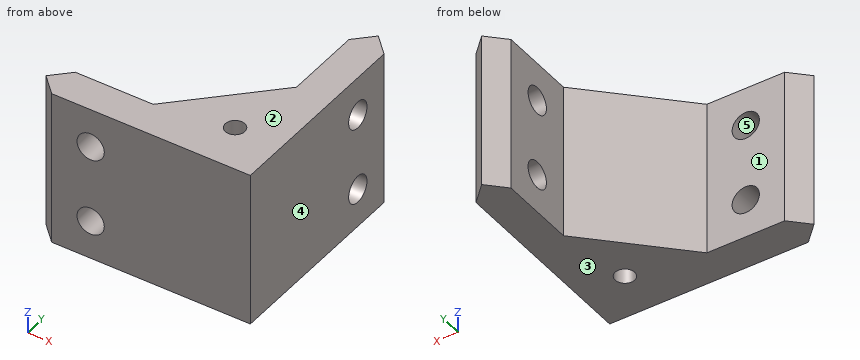
from build123d import *

# Parameters (mm, degrees)
BOSS_EXTRUDE1_DEPTH = 40
SKETCH2_R           = 3.5
CUT_EXTRUDE1_DEPTH  = 84.3366666
SKETCH3_R           = 3.5
CUT_EXTRUDE2_DEPTH  = 40
CHAMFER1_SIZE       = 5
SKETCH4_R           = 2.5
CUT_EXTRUDE3_DEPTH  = 40


with BuildPart() as part:
    # Sketch1 → Boss-Extrude1 (new body)
    with BuildSketch(Plane.XY):
        Polygon((0, 56), (0, 0), (-56, 0), (-56, 9), (-31, 9), (-9, 31), (-9, 56), align=None)
    extrude(amount=BOSS_EXTRUDE1_DEPTH)

    # Sketch2 → Cut-Extrude1 (cut, through all)
    with BuildSketch(Plane.ZY.offset(9)):
        with Locations((10, 41)):
            Circle(SKETCH2_R)
        with Locations((30, 41)):
            Circle(SKETCH2_R)
    extrude(amount=-CUT_EXTRUDE1_DEPTH, mode=Mode.SUBTRACT)

    # Sketch3 → Cut-Extrude2 (cut)
    with BuildSketch(Plane(origin=(0, 9, 0), x_dir=(1, 0, 0), z_dir=(0, 1, 0))):
        with Locations(Location((-41, -10, 0), (0, 0, 270))):
            Circle(SKETCH3_R)
        with Locations(Location((-41, -30, 0), (0, 0, 270))):
            Circle(SKETCH3_R)
    extrude(amount=-CUT_EXTRUDE2_DEPTH, mode=Mode.SUBTRACT)

    # Chamfer1
    # the kernel refuses this chamfer: 5 mm, written as the material it takes off along each edge
    with BuildSketch(Plane(origin=(-56, 0, -12.85841494), x_dir=(0.9996219169112968, -0.027495876610586254, 0), z_dir=(0, 0, 1)), Plane(origin=(-56, 9, -12.85841494), x_dir=(-0.027495876610586317, -0.9996219169112968, 0), z_dir=(0, 0, 1))) as chamfer1_piece_1:
        Polygon((CHAMFER1_SIZE * 0.999621916911, CHAMFER1_SIZE * 0.0274958766106), (-CHAMFER1_SIZE * 0.0274958766106, CHAMFER1_SIZE * 0.999621916911), (0, 0), align=None)
    extrude(amount=65.71682988, mode=Mode.SUBTRACT)
    with BuildSketch(Plane(origin=(0, 56, -12.85841494), x_dir=(0.02749587661058641, -0.9996219169112968, 0), z_dir=(0, 0, 1)), Plane(origin=(-9, 56, -12.85841494), x_dir=(0.9996219169112968, 0.027495876610586317, 0), z_dir=(0, 0, 1))) as chamfer1_piece_2:
        Polygon((CHAMFER1_SIZE * 0.999621916911, -CHAMFER1_SIZE * 0.0274958766106), (-CHAMFER1_SIZE * 0.0274958766106, -CHAMFER1_SIZE * 0.999621916911), (0, 0), align=None)
    extrude(amount=65.71682988, mode=Mode.SUBTRACT)

    # Sketch4 → Cut-Extrude3 (cut)
    with BuildSketch(Plane(origin=(0, 0, 0), x_dir=(-1, 0, 0), z_dir=(0, 0, -1))):
        with Locations((12, 12)):
            Circle(SKETCH4_R)
    extrude(amount=-CUT_EXTRUDE3_DEPTH, mode=Mode.SUBTRACT)


solid = part.part
The listing builds one solid part. Answer for the finished solid, in the listing's coordinates (mm). Face numbers are marked on the shaded views. A direction names the side the tool comes from. Give positions to 0.01 mm unless a question says otherwise; leave off trailing zeros. Loops run counter-clockwise (first coordinate to the right, second up) from the corner with the lowest first, then second, coordinate; pieces in that order, holes last. Notation, with made-up numbers: (-34.5, 64) - (8.5, 64) arc R30 ccw to (8.5, 90) - close; hole circle Ø2 at (15, -36). An arc over 180 degrees is marked (long way). Write each question's results on one line, items separated by ' | '.
1. Flat-ended cylindrical pins translate along their axes: P1, Ø6, axis at y = 39, z = 29, coming from the -X side; P2, Ø4, axis at y = 41, z = 10, coming from the -X side; P3, Ø16, axis at x = -36.5, z = 13.5, coming from the +Y side; P4, Ø3, axis at y = 19, z = 29.5, coming from the -X side. Find the tip coordinate at first contact, or state that the pin passes through.
Resolved:
P1: stops at x = -9 | P2: passes through | P3: stops at y = 11.5 | P4: stops at x = -22.5
2. Find section D-D, the plane y = 41. Write down the section's boundary in (x, z), then the cut area to 3 significant figures.
Resolved:
outline: (-9, 0) - (0, 0) - (0, 6.5) - (-9, 6.5) - close; (-9, 13.5) - (0, 13.5) - (0, 26.5) - (-9, 26.5) - close; (-9, 33.5) - (0, 33.5) - (0, 40) - (-9, 40) - close | area: 234 mm^2
3. Find section C-C, the plane x = -13.5. Write down the section's boundary in (y, z), then the cut area to 3 significant figures.
Resolved:
outline: (0, 0) - (10, 0) - (10, 40) - (0, 40) - close; (14, 0) - (26.5, 0) - (26.5, 40) - (14, 40) - close | area: 900 mm^2
4. Find section B-B, the plane y = 12. Write down the section's boundary in (x, z).
Resolved:
outline: (-28, 0) - (-14.5, 0) - (-14.5, 40) - (-28, 40) - close; (-9.5, 0) - (0, 0) - (0, 40) - (-9.5, 40) - close
5. Consider probe 1 along X at (y, z) = (47.5, 13.5); probe 2 along X at (y, z) = (4, 12.5); probe 3 along Y at (x, z) = (-42, 21.5). Determine where each line is inside the solid, lowest interval first. Write a range as from..to.
Resolved:
probe 1: x = -9..0 | probe 2: x = -55..-43.45, -38.55..0 | probe 3: y = 0..9
6. Find section A-A, the plane z = 10. Write down the section's boundary in (x, y).
Resolved:
outline: (-55.5, 4.5) - (-51, 0) - (-44.5, 0) - (-44.5, 9) - (-51, 9) - close; (-37.5, 0) - (0, 0) - (0, 37.5) - (-9, 37.5) - (-9, 31) - (-31, 9) - (-37.5, 9) - close; (-9, 44.5) - (0, 44.5) - (0, 51) - (-4.5, 55.5) - (-9, 51) - close; hole circle Ø5 at (-12, 12)
7. Which of the six approach directions +Z, -Z, +X, -X, +Y, -Y give full straight-line access (tool end or side, diameter ignored) to the marked faces 1 and 2?
Resolved:
face 1: +Z, -Z, -X, +Y | face 2: +Z, +X, -X, +Y, -Y
8. For a pull along X with two mould halves and no side action, classify the marked faces 3, 4 and 5 as +X half, -X half, draft (parallel to the pull), parting line (faces both ways), or undercut.
Resolved:
face 3: draft | face 4: +X half | face 5: undercut
